Check sheet for the modelled part. Datum: model origin and axes. Units: mm. A direction names the side the tool comes from. Give positions to 0.01 mm unless a question says otherwise; leave off trailing zeros. Loops run counter-clockwise (first coordinate to the right, second up) from the corner with the lowest first, then second, coordinate; pieces in that order, holes last. Notation, with made-up numbers: M 27,15 L 74,15 A15 cw 74,24 Z; hole C 54,88.25 d5. An arc over 180 degrees is marked long. One line per question, with ' | ' between items. Start each with the question number.
from build123d import *

# Parameters (mm, degrees)
SKETCH_1_W          = 15
SKETCH_1_H          = 15
EXTRUDE_1_DEPTH     = 5
SKETCH_2_R          = 1.5
SKETCH_2_R_2        = 1.25
SKETCH_2_R_3        = 2.8
SKETCH_2_R_4        = 1
CUT_EXTRUDE_1_DEPTH = 5
FILLET_1_R          = 1.5
SKETCH_4_R          = 1.5
EXTRUDE_2_DEPTH     = 2
SKETCH_5_R          = 2
CUT_EXTRUDE_2_DEPTH = 5
CUT_EXTRUDE_3_DEPTH = 5


with BuildPart() as part:
    # 草图1 → 凸台-拉伸1 (new body)
    with BuildSketch(Plane(origin=(0, 0, 0), x_dir=(1, 0, 0), z_dir=(0, 1, 0))):
        Polygon((30, 16), (-30, 16), (-30, -1), (-30, -16), (30, -16), align=None)
        with Locations((-37.5, -8.5)):
            Rectangle(SKETCH_1_W, SKETCH_1_H)
    extrude(amount=EXTRUDE_1_DEPTH)

    # 草图2 → 切除-拉伸1 (cut)
    with BuildSketch(Plane(origin=(0, 5, 0), x_dir=(1, 0, 0), z_dir=(0, 1, 0))):
        with Locations(Location((8.5, 0, 0), (0, 0, 270))):
            Circle(SKETCH_2_R)
        with Locations(Location((-8.5, 0, 0), (0, 0, 90))):
            Circle(SKETCH_2_R)
        with Locations(Location((0, 0, 0), (0, 0, 270))):
            Circle(SKETCH_2_R_2)
        with Locations(Location((20, 0, 0), (0, 0, 270))):
            Circle(SKETCH_2_R_3)
        with Locations(Location((-20, 0, 0), (0, 0, 90))):
            Circle(SKETCH_2_R_3)
        with Locations(Location((20, 8, 0), (0, 0, 270))):
            Circle(SKETCH_2_R_2)
        with Locations(Location((28, 0, 0), (0, 0, 270))):
            Circle(SKETCH_2_R_2)
        with Locations(Location((-28, 0, 0), (0, 0, 90))):
            Circle(SKETCH_2_R_2)
        with Locations(Location((-20, 8, 0), (0, 0, 90))):
            Circle(SKETCH_2_R_2)
        with Locations(Location((-37.5, -8.5, 0), (0, 0, 270))):
            Circle(SKETCH_2_R)
        with Locations(Location((-32, -8.5, 0), (0, 0, 270))):
            Circle(SKETCH_2_R_4)
        with Locations(Location((-37.5, -14, 0), (0, 0, 270))):
            Circle(SKETCH_2_R_4)
        with Locations(Location((-43, -8.5, 0), (0, 0, 270))):
            Circle(SKETCH_2_R_4)
        with Locations(Location((-37.5, -3, 0), (0, 0, 270))):
            Circle(SKETCH_2_R_4)
    extrude(amount=-CUT_EXTRUDE_1_DEPTH, mode=Mode.SUBTRACT)

    # 圆角1
    fillet_1_edges = [part.edges().sort_by_distance(p)[0] for p in [
        (-30, 2.5, 1),
        (-45, 2.5, 1),
        (-30, 2.5, -16),
        (30, 2.5, -16),
    ]]
    fillet(fillet_1_edges, radius=FILLET_1_R)

    # 草图4 → 凸台-拉伸2 (add)
    with BuildSketch(Plane.XY.offset(16)):
        with Locations(Location((20, 2.5, 0), (0, 0, 180))):
            Circle(SKETCH_4_R)
        with Locations(Location((-20, 2.5, 0), (0, 0, 180))):
            Circle(SKETCH_4_R)
    extrude(amount=EXTRUDE_2_DEPTH)

    # 草图5 → 切除-拉伸2 (cut)
    with BuildSketch(Plane(origin=(0, 0, -16), x_dir=(-1, 0, 0), z_dir=(0, 0, -1))):
        with Locations((-20, 2.5)):
            Circle(SKETCH_5_R)
        with Locations(Location((20, 2.5, 0), (0, 0, 180))):
            Circle(SKETCH_5_R)
    extrude(amount=-CUT_EXTRUDE_2_DEPTH, mode=Mode.SUBTRACT)

    # 草图6 → 切除-拉伸3 (cut)
    with BuildSketch(Plane.XZ):
        with BuildLine():
            Line((-25, 14.5), (25, 14.5))
            ThreePointArc((25, 14.5), (26, 13.5), (25, 12.5))
            Line((25, 12.5), (-25, 12.5))
            ThreePointArc((-25, 12.5), (-26, 13.5), (-25, 14.5))
        make_face()
        with BuildLine():
            Line((-25, 11.7), (25, 11.7))
            ThreePointArc((25, 11.7), (26, 10.7), (25, 9.7))
            Line((25, 9.7), (-25, 9.7))
            ThreePointArc((-25, 9.7), (-26, 10.7), (-25, 11.7))
        make_face()
        with BuildLine():
            Line((-25, 8.9), (25, 8.9))
            ThreePointArc((25, 8.9), (26, 7.9), (25, 6.9))
            Line((25, 6.9), (-25, 6.9))
            ThreePointArc((-25, 6.9), (-26, 7.9), (-25, 8.9))
        make_face()
        with BuildLine():
            Line((-25, 6.1), (25, 6.1))
            ThreePointArc((25, 6.1), (26, 5.1), (25, 4.1))
            Line((25, 4.1), (-25, 4.1))
            ThreePointArc((-25, 4.1), (-26, 5.1), (-25, 6.1))
        make_face()
        with BuildLine():
            Line((-16, -2.4), (16, -2.4))
            ThreePointArc((16, -2.4), (17.2, -3.6), (16, -4.8))
            Line((16, -4.8), (-16, -4.8))
            ThreePointArc((-16, -4.8), (-17.2, -3.6), (-16, -2.4))
        make_face()
        with BuildLine():
            Line((-14, -5.6), (14, -5.6))
            ThreePointArc((14, -5.6), (15.2, -6.8), (14, -8))
            Line((14, -8), (-14, -8))
            ThreePointArc((-14, -8), (-15.2, -6.8), (-14, -5.6))
        make_face()
        with BuildLine():
            Line((-14, -8.8), (14, -8.8))
            ThreePointArc((14, -8.8), (15.2, -10), (14, -11.2))
            Line((14, -11.2), (-14, -11.2))
            ThreePointArc((-14, -11.2), (-15.2, -10), (-14, -8.8))
        make_face()
        with BuildLine():
            Line((-14, -12), (14, -12))
            ThreePointArc((14, -12), (15.2, -13.2), (14, -14.4))
            Line((14, -14.4), (-14, -14.4))
            ThreePointArc((-14, -14.4), (-15.2, -13.2), (-14, -12))
        make_face()
        with BuildLine():
            Line((-22.3, -4), (-22.3, -12))
            ThreePointArc((-22.3, -12), (-23.5, -13.2), (-24.7, -12))
            Line((-24.7, -12), (-24.7, -4))
            ThreePointArc((-24.7, -4), (-23.5, -2.8), (-22.3, -4))
        make_face()
        with BuildLine():
            Line((-26.3, -4), (-26.3, -12))
            ThreePointArc((-26.3, -12), (-27.5, -13.2), (-28.7, -12))
            Line((-28.7, -12), (-28.7, -4))
            ThreePointArc((-28.7, -4), (-27.5, -2.8), (-26.3, -4))
        make_face()
        with BuildLine():
            Line((22.3, -4), (22.3, -12))
            ThreePointArc((22.3, -12), (23.5, -13.2), (24.7, -12))
            Line((24.7, -12), (24.7, -4))
            ThreePointArc((24.7, -4), (23.5, -2.8), (22.3, -4))
        make_face()
        with BuildLine():
            Line((26.3, -4), (26.3, -12))
            ThreePointArc((26.3, -12), (27.5, -13.2), (28.7, -12))
            Line((28.7, -12), (28.7, -4))
            ThreePointArc((28.7, -4), (27.5, -2.8), (26.3, -4))
        make_face()
    extrude(amount=-CUT_EXTRUDE_3_DEPTH, mode=Mode.SUBTRACT)


solid = part.part
Q1. Material ranges on probe 1 along Y at (x, z) = (20, -12); probe 2 along X at (y, z) = (3.5, 8.5); probe 3 along Z at (x, y) = (-17, 2.35), recorded low to high. Write a range as from..to.
Q2. Cross-section at B-B (x = -2.5). State how many separate pieces and enclosed holes the cut face has, and give its area (3 significant figures).
Q3. Depth check by flat-ended pin: P1, Ø1.5, axis at y = 1.5, z = -6, coming from the -X side; P2, Ø2.5, axis at x = -1.5, y = 3.5, coming from the +Z side; P3, Ø1.2, axis at x = -19, y = 2.5, coming from the -Z side. Enter the tip coordinate at first touch or a pass-through.
Q4. Cross-section at A-A (x = 23.5). Record the cut outline in (y, z).
Q5. Draft check along X on faces 4 (the cylindrical face through (-23.5, 2.5, -13.2)), 5 (the cylindrical face through (-23.5, 2.5, -2.8)), 6 (the flat face through (-20, 2, 18)), 7 (the cylindrical face through (29.55, 2.54, -15.57)). Enter one of: released by +X, released by -X, zero draft, split by the parting line, or undercut.
Q6. Access from +Z, -Z, +X, -X, +Y, -Y to the whole of each face (thin tool, end or side, straight path). Record for faces 1 (the flat face through (-20, 2, -11)), 2 (the cylindrical face through (-29.55, 2.54, -15.57)), 3 (the cylindrical face through (15.2, 2.5, -6.8)).
Solved:
1) probe 1: y = 0..0.5, 4.5..5 | probe 2: x = -45..-44, -42..-39, -36..-33, -31..-25.8, 25.8..30 | probe 3: z = -16..-4.26, -2.94..4.1, 6.1..6.9, 8.9..9.7, 11.7..12.5, 14.5..16
2) separate pieces: 9 | enclosed holes: 0 | area: 72.0 mm²
3) P1: stops at x = -30 | P2: stops at z = 16 | P3: stops at z = -11
4) outline: M 0,-16 L 5,-16 L 5,-13.2 L 0,-13.2 Z; M 0,-2.8 L 5,-2.8 L 5,4.1 L 0,4.1 Z; M 0,6.1 L 5,6.1 L 5,6.9 L 0,6.9 Z; M 0,8.9 L 5,8.9 L 5,9.7 L 0,9.7 Z; M 0,11.7 L 5,11.7 L 5,12.5 L 0,12.5 Z; M 0,14.5 L 5,14.5 L 5,16 L 0,16 Z
5) face 4: undercut | face 5: undercut | face 6: zero draft | face 7: released by +X
6) face 1: -Z | face 2: -Z, -X, +Y, -Y | face 3: +Y, -Y
